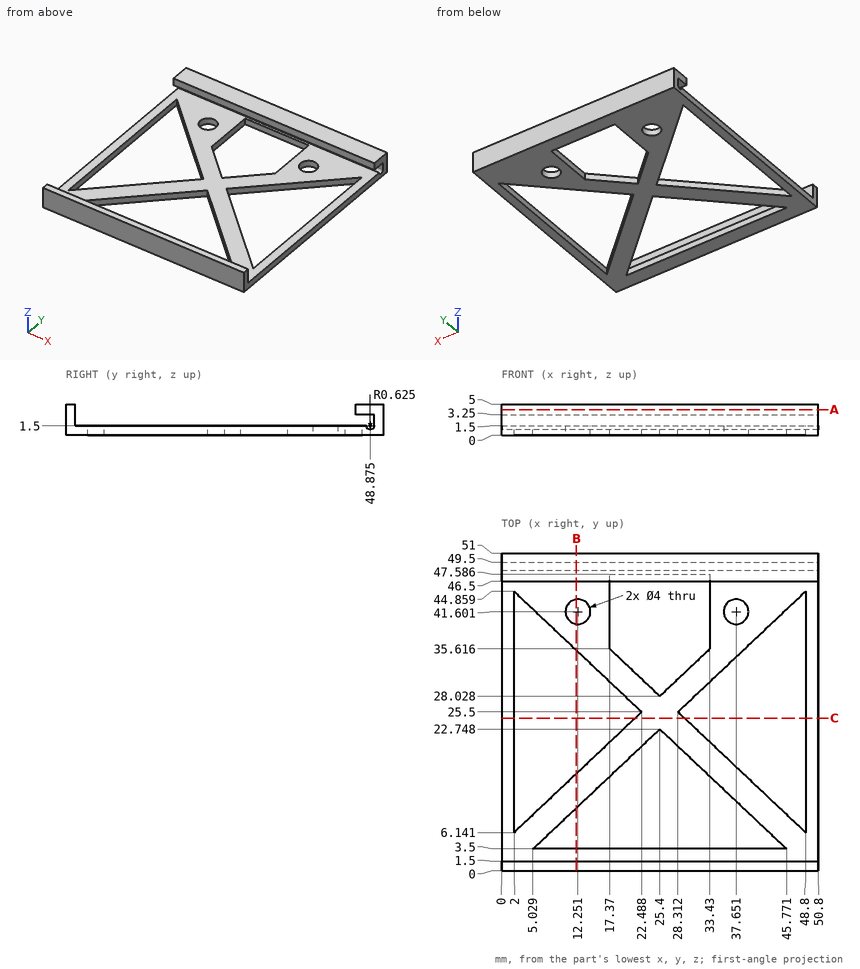
Study the drawing (mm; zero at the part's minimum x, y, z) and answer. Give positions to 0.01 mm unless a question says otherwise; leave off trailing zeros. Order: outer loops, then holes, each group sorted by start corner. A loop starts at its lowest first (then second) coordinate and runs counter-clockwise, first axis right, second up. Notation, with made-up numbers: (43.5, 2) -> (61.5, 2) arc R23 ccw to (61.5, 41) -> close; hole circle Ø11 at (12, -3.5). An arc over 180 degrees is marked (long way). Put each result on its own line as item: value.
Item 1: Given P1, Ø5, axis at x = 37.65, y = 41.6, coming from the +Z side; P2, Ø2, axis at x = 29, y = 17.5, coming from the -Z side, each flat-ended and moving along its own axis, determine where each tip first touches the part or whether it passes through.
Established:
P1: stops at z = 1.5
P2: passes through
Item 2: A cutting plane is placed at A-A on z = 4.1. Give the vertices of the cut face in (x, y).
Established:
outline: (0, 0) -> (50.8, 0) -> (50.8, 1.5) -> (0, 1.5) -> close; (0, 46.5) -> (50.8, 46.5) -> (50.8, 51) -> (0, 51) -> close
Item 3: Straight lines are drawn through the part: line 1 (X direction, y = 37.5, z = 0.65) (1 decimal); line 2 (Y direction, x = 28, z = 3.05); line 3 (Y direction, x = 46.5, z = 4.4). For each, find the intervals that lie inside material, in ascending order.
Established:
line 1: x = 0 to 2, 9.8 to 17.4, 33.4 to 41, 48.8 to 50.8
line 2: y = 0 to 1.5, 49.5 to 51
line 3: y = 0 to 1.5, 46.5 to 51
Item 4: A cutting plane is placed at B-B on x = 12. Count the separate pieces of the cut face and the enclosed holes in it.
Established:
separate pieces: 4
enclosed holes: 0
Item 5: A cutting plane is placed at C-C on y = 24.5. Give the vertices of the cut face in (x, z), plus the area to 3 significant figures.
Established:
outline: (0, 0) -> (2, 0) -> (2, 1.5) -> (0, 1.5) -> close; (21.43, 0) -> (29.37, 0) -> (29.37, 1.5) -> (21.43, 1.5) -> close; (48.8, 0) -> (50.8, 0) -> (50.8, 1.5) -> (48.8, 1.5) -> close
area: 17.9 mm^2
